Check sheet for the modelled part. Datum: model origin and axes. Units: mm. Face numbers are marked on the shaded views. Give positions to 0.01 mm unless a question says otherwise; leave off trailing zeros. Order: outer loops, then holes, each group sorted by start corner. A loop starts at its lowest first (then second) coordinate and runs counter-clockwise, first axis right, second up. Notation, with made-up numbers: M 77,-6 L 132,-6 A18 ccw 132,22 Z; hole C 88,42.25 d11. An arc over 180 degrees is marked long. One line per question, with ' | ' between items. Start each with the question number.
```python
from build123d import *

# Parameters (mm, degrees)
F0_R     = 1.75
F1_DEPTH = 8
F2_R     = 1.75
F3_DEPTH = 20


with BuildPart() as f1:
    # F0 (on Top) → F1 (new body)
    with BuildSketch(Plane.XY):
        with BuildLine():
            Line((-4, 16), (-4, 0))
            ThreePointArc((-4, 0), (0, -4), (4, 0))
            Line((4, 0), (4, 16))
            Line((4, 16), (-4, 16))
        make_face()
        Circle(F0_R, mode=Mode.SUBTRACT)
    extrude(amount=F1_DEPTH)

    # F2 (on face) → F3 (cut)
    with BuildSketch(Plane.YZ.offset(4)):
        with Locations((12.5, 4)):
            Circle(F2_R)
    extrude(amount=-F3_DEPTH, mode=Mode.SUBTRACT)


solid = f1.part
```
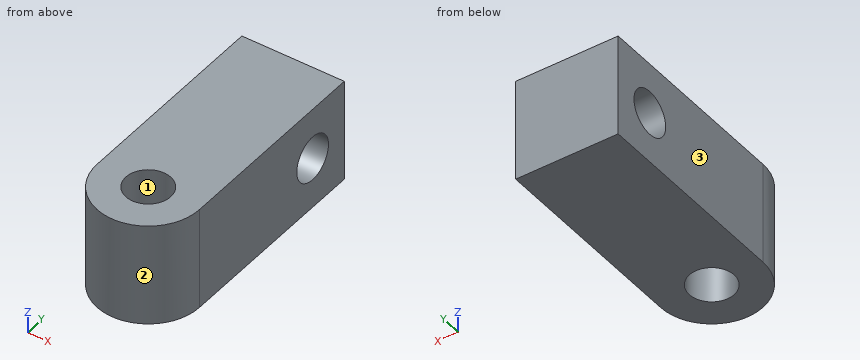
Item 1: Section check B-B, the plane x = 0. Record the cut outline in (y, z), then the cut area to 3 significant figures.
Item 2: Section check A-A, the plane z = 4. Record the cut outline in (x, y).
Item 3: Draft check along Y on the marked faces 1, 2 and 3. Enter one of: released by +Y, released by -Y, zero draft, split by the parting line, or undercut.
Item 4: Section check D-D, the plane z = 7.75. Record the cut outline in (x, y).
Item 5: Scan lines: probe 1 along Y at (x, z) = (0, 5); probe 2 along Z at (x, y) = (-1.75, 12.5); probe 3 along Y at (x, z) = (0, 4.5). Record each from-to range of solid material in increasing order. Write a range as [from, to].
Item 6: Section check C-C, the plane y = 12.5. Record the cut outline in (x, z), then the cut area to 3 significant figures.
Reported:
1) outline: M -4,0 L -1.75,0 L -1.75,8 L -4,8 Z; M 1.75,0 L 16,0 L 16,8 L 1.75,8 Z; hole C 12.5,4 d3.5 | area: 122 mm^2
2) outline: M -4,0 A4 ccw 4,0 L 4,10.75 L -4,10.75 Z; M -4,14.25 L 4,14.25 L 4,16 L -4,16 Z; hole C 0,0 d3.5
3) face 1: undercut | face 2: released by -Y | face 3: zero draft
4) outline: M -4,0 A4 ccw 4,0 L 4,16 L -4,16 Z; hole C 0,0 d3.5
5) probe 1: y = [-4, -1.75], [1.75, 11.06], [13.94, 16] | probe 2: z = [0, 2.25], [5.75, 8] | probe 3: y = [-4, -1.75], [1.75, 10.82], [14.18, 16]
6) outline: M -4,0 L 4,0 L 4,2.25 L -4,2.25 Z; M -4,5.75 L 4,5.75 L 4,8 L -4,8 Z | area: 36.0 mm^2
